Check sheet for the modelled part. Datum: model origin and axes. Units: mm. Face numbers are marked on the shaded views. A direction names the side the tool comes from. Coordinates: 2 decimals unless noted, no trailing zeros. Write each loop counter-clockwise with the first axis right and the second up, starting at its lowest first coordinate (ties: lowest second). Pieces come first, ordered by that corner, then holes. Notation, with made-up numbers: (41.5, 83.5) -> (60.5, 83.5) arc R22 cw to (60.5, 104.5) -> close; hole circle Ø4 at (59, -30.75). An arc over 180 degrees is marked (long way). One line per item, written item: value. Start each with the question number.
1) Set-up check for the marked faces 1, 2 and 3: record each of +Z, -Z, +X, -X, +Y, -Y from which the full face is reachable in a straight line by a thin tool's end or side.
2) Scan lines: line 1 along Z through (x, y) = (-59.85, 13.75); line 2 along X through (y, z) = (6.5, -52.18); line 3 along X through (y, z) = (13.75, -9). Record each from-to range of solid material in increasing order. Write a range as [from, to].
3) Gauge pin test, flat ends, axial feed: P1, Ø1.5, axis at x = -15.5, y = 15, coming from the +Z side; P2, Ø9, axis at x = -5.7, z = -9, coming from the +Y side; P3, Ø2.5, axis at x = -6, z = -8, coming from the +Y side; P4, Ø3, axis at x = -50.5, y = 34, coming from the +Z side. Record the tip position at first contact, or that the pin passes through.
4) Sectioned sample at B-B on y = 12.5. Enter the section's corners in (x, z).
5) Sectioned sample at C-C on x = -5.7. Enter the section's corners in (y, z).
6) Sectioned sample at A-A on z = -2.5. Enter the section's corners in (x, y).
7) Sectioned sample at D-D on z = -9. Enter the section's corners in (x, y).
Autodesk Inventor part; units mm, degrees
ref_plane "YZ Plane" through (0, 0, 0) normal (1, 0, 0) x (0, 1, 0)
ref_plane "XZ Plane" through (0, 0, 0) normal (0, 1, 0) x (-1, 0, 0)
ref_plane "XY Plane" through (0, 0, 0) normal (0, 0, 1) x (1, 0, 0)
sketch "Sketch1" plane through (0, 0, 0) normal (0, 1, 0) x (-1, 0, 0)
  line L0 (0, 0) -> (62.35, 0)
  line L1 (62.35, 0) -> (62.35, -54.68)
  line L2 (62.35, -54.68) -> (0, -54.68)
  line L3 (0, -54.68) -> (0, 0)
  dimension "d0" = 54.68
  dimension "d1" = 62.35
extrude "Extrusion1" add sketch "Sketch1" along normal blind 19
sketch "Sketch2" plane through (0, 19, 0) normal (0, 1, 0) x (1, 0, 0)
  line L0 (-62.35, 54.68) -> (-62.35, 0)
  line L1 (0, 54.68) -> (-62.35, 54.68)
  point P0 (0, 0)
  point P1 (-59.85, 52.18)
  dimension "d4" = 2.5
  dimension "d5" = 2.5
hole "Hole1" at (-59.85, 19, -52.18) direction (0, -1, 0) diameter 3 end through all
ref_plane "Work Plane1" through (-62.35, 0, -27.34) normal (0, 0, 1) x (1, 0, 0)
ref_plane "Work Plane2" through (-31.175, 0, 0) normal (1, 0, 0) x (0, 0, -1)
mirror "Mirror1" about plane through (-62.35, 0, -27.34) normal (0, 0, 1) of "Hole1"
mirror "Mirror2" about plane through (-31.175, 0, 0) normal (1, 0, 0) of "Hole1", "Mirror1"
sketch "Sketch3" plane through (0, 19, 0) normal (0, 1, 0) x (1, 0, 0)
  line L0 (-48.05, 1) -> (-52.05, 1)
  line L1 (-52.05, 1) -> (-52.05, 17.4)
  line L2 (-52.05, 17.4) -> (-48.05, 17.4)
  line L3 (-48.05, 17.4) -> (-48.05, 1)
  line L4 (-62.35, 0) -> (0, 0)
  line L5 (-62.35, 54.68) -> (-62.35, 0)
  dimension "d13" = 4
  dimension "d14" = 16.4
  dimension "d15" = 1
  dimension "d16" = 10.3
extrude "Extrusion2" add sketch "Sketch3" along normal blind 28.6
sketch "Sketch4" plane through (0, 19, 0) normal (0, 1, 0) x (1, 0, 0)
  circle A0 centre (-5.7, 9) radius 2.75
  line L0 (-62.35, 0) -> (0, 0)
  line L1 (0, 0) -> (0, 54.68)
  dimension "d19" = 5.5
  dimension "d20" = 9
  dimension "d21" = 5.7
extrude "Extrusion3" cut sketch "Sketch4" against normal blind 10
properties part number "board"
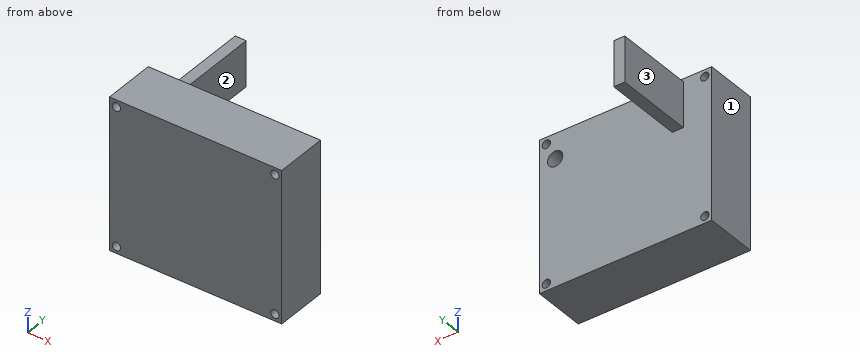
Answers:
1. face 1: +Z, -Z, -X, +Y, -Y
1. face 2: +Z, -Z, +X, +Y
1. face 3: +Z, -Z, -X, +Y
2. line 1: z = [-54.68, -53.68], [-50.68, -4], [-1, 0]
2. line 2: x = [-62.35, -61.35], [-58.35, -4], [-1, 0]
2. line 3: x = [-62.35, -8.45], [-2.95, 0]
3. P1: stops at z = 0
3. P2: stops at y = 19
3. P3: stops at y = 9
3. P4: stops at z = -1
4. outline: (-62.35, -54.68) -> (0, -54.68) -> (0, 0) -> (-62.35, 0) -> close; hole circle Ø3 at (-59.85, -52.18); hole circle Ø3 at (-59.85, -2.5); hole circle Ø5.5 at (-5.7, -9); hole circle Ø3 at (-2.5, -52.18); hole circle Ø3 at (-2.5, -2.5)
5. outline: (0, -54.68) -> (19, -54.68) -> (19, -11.75) -> (9, -11.75) -> (9, -6.25) -> (19, -6.25) -> (19, 0) -> (0, 0) -> close
6. outline: (-62.35, 0) -> (-61.35, 0) -> (-61.35, 19) -> (-62.35, 19) -> close; (-58.35, 0) -> (-4, 0) -> (-4, 19) -> (-48.05, 19) -> (-48.05, 47.6) -> (-52.05, 47.6) -> (-52.05, 19) -> (-58.35, 19) -> close; (-1, 0) -> (0, 0) -> (0, 19) -> (-1, 19) -> close
7. outline: (-62.35, 0) -> (0, 0) -> (0, 19) -> (-2.95, 19) -> (-2.95, 9) -> (-8.45, 9) -> (-8.45, 19) -> (-48.05, 19) -> (-48.05, 47.6) -> (-52.05, 47.6) -> (-52.05, 19) -> (-62.35, 19) -> close
